from build123d import *

# Parameters (mm, degrees)
ESQUISSE4_W             = 100
ESQUISSE4_H             = 100
ESQUISSE4_W_2           = 90
ESQUISSE4_H_2           = 90
BOSS_EXTRU_1_DEPTH      = 100
ESQUISSE5_W             = 100
ESQUISSE5_H             = 100
BOSS_EXTRU_2_DEPTH      = 10
ESQUISSE6_W             = 95
ESQUISSE6_H             = 94.999780415
ENL_V_MAT_EXTRU_1_DEPTH = 95
ESQUISSE7_W             = 95
ESQUISSE7_H             = 95
ENL_V_MAT_EXTRU_2_DEPTH = 1
ESQUISSE8_W             = 95
ESQUISSE8_H             = 95
BOSS_EXTRU_3_DEPTH      = 1
ENL_V_MAT_EXTRU_4_DEPTH = 55.5
ENL_V_MAT_EXTRU_5_DEPTH = 21.5


with BuildPart() as part:
    # Esquisse4 → Boss.-Extru.1 (new body)
    with BuildSketch(Plane.XY):
        with Locations((1.564199822, -3.801871506)):
            Rectangle(ESQUISSE4_W, ESQUISSE4_H)
        with Locations((1.564199822, -3.801871506)):
            Rectangle(ESQUISSE4_W_2, ESQUISSE4_H_2, mode=Mode.SUBTRACT)
    extrude(amount=BOSS_EXTRU_1_DEPTH)

    # Esquisse5 → Boss.-Extru.2 (add)
    with BuildSketch(Plane.XY.offset(100)):
        with Locations((1.564199822, -3.801871506)):
            Rectangle(ESQUISSE5_W, ESQUISSE5_H)
    extrude(amount=-BOSS_EXTRU_2_DEPTH)

    # Esquisse6 → Enlèv. mat.-Extru.1 (cut)
    with BuildSketch(Plane(origin=(0, 0, 0), x_dir=(-1, 0, 0), z_dir=(0, 0, -1))):
        with Locations((0.935800178, -1.301761713)):
            Rectangle(ESQUISSE6_W, ESQUISSE6_H)
    extrude(amount=-ENL_V_MAT_EXTRU_1_DEPTH, mode=Mode.SUBTRACT)

    # Esquisse7 → Enlèv. mat.-Extru.2 (cut)
    with BuildSketch(Plane(origin=(0, -48.801651921, 0), x_dir=(1, 0, 0), z_dir=(0, 1, 0))):
        with Locations((-0.935800178, -47.5)):
            Rectangle(ESQUISSE7_W, ESQUISSE7_H)
    extrude(amount=-ENL_V_MAT_EXTRU_2_DEPTH, mode=Mode.SUBTRACT)

    # Esquisse8 → Boss.-Extru.3 (add)
    with BuildSketch(Plane(origin=(0, -49.801651921, 0), x_dir=(1, 0, 0), z_dir=(0, 1, 0))):
        with Locations((-0.935800178, -47.5)):
            Rectangle(ESQUISSE8_W, ESQUISSE8_H)
    extrude(amount=BOSS_EXTRU_3_DEPTH)

    # Esquisse9 → Enlèv. mat.-Extru.4 (cut)
    with BuildSketch(Plane(origin=(0, 0, 95), x_dir=(-1, 0, 0), z_dir=(0, 0, -1))):
        with BuildLine():
            ThreePointArc((23.184567711, 20.946945437), (-26.312906972, 20.94700582), (-26.312967355, -28.550468863))
            Line((-26.312967355, -28.550468863), (23.184567711, 20.946945437))
        make_face()
        with BuildLine():
            Line((23.184567711, 20.946945437), (-26.312967355, -28.550468863))
            ThreePointArc((-26.312967355, -28.550468863), (11.829700587, -36.137553521), (33.435800178, -3.801761713))
            ThreePointArc((33.435800178, -3.801761713), (30.771591985, 9.592138696), (23.184567711, 20.946945437))
        make_face()
    extrude(amount=-ENL_V_MAT_EXTRU_4_DEPTH, mode=Mode.SUBTRACT)

    # Esquisse11 → Enlèv. mat.-Extru.5 (cut)
    with BuildSketch(Plane.ZY.offset(-46.564199822)):
        with BuildLine():
            ThreePointArc((25.251232467, 20.946945437), (25.25129285, -28.550529246), (74.748767533, -28.550468863))
            Line((74.748767533, -28.550468863), (25.251232467, 20.946945437))
        make_face()
        with BuildLine():
            Line((25.251232467, 20.946945437), (74.748767533, -28.550468863))
            ThreePointArc((74.748767533, -28.550468863), (82.335791808, -17.195662123), (85, -3.801761713))
            ThreePointArc((85, -3.801761713), (63.393900409, 28.534030094), (25.251232467, 20.946945437))
        make_face()
    extrude(amount=-ENL_V_MAT_EXTRU_5_DEPTH, mode=Mode.SUBTRACT)


solid = part.part
Design review of the part built by this model. Coordinates are the model's own, in mm. A direction names the side the tool comes from. Round coordinates to 2 decimals unless told otherwise and drop trailing zeros. Write each loop counter-clockwise with the first axis right and the second up, starting at its lowest first coordinate (ties: lowest second). Pieces come first, ordered by that corner, then holes.
Item 1: Consider section D-D on x = -35. Give the boundary of the cut face in (y, z), and give its area (3 significant figures).
Item 2: For faces 1 (the flat face through (-2, -48.802, 47)), 2 (the flat face through (-48.436, -26, 98)), list the 3-axis set-ups (+Z, -Z, +X, -X, +Y, -Y) from which the entire face can be reached by the end or side of a thin tool; tool diameter is ignored.
Item 3: Wall thickness on L1, parallel to Z at x = 1.5, y = 31.5; L2, parallel to Y at x = -32.5, z = 37; L3, parallel to X at y = 37, z = 64: over which ranges is each line inside the solid? List them lowest first.
Item 4: Consider section C-C on x = 8. Give the boundary of the cut face in (y, z), and give its area (3 significant figures).
Item 5: Consider section B-B on y = 15. Give the boundary of the cut face in (x, z), and give its area (3 significant figures).
Item 6: For pin 1 Ø3 at (y, z) = (-17, 20.5) entering from -X; pin 2 Ø8 at (x, z) = (-10, 89) entering from +Y; pin 3 Ø12 at (y, z) = (13, 74) entering from -X, all flat-tipped, find the tip position at first contact; note any pin that passes through.
Item 7: Consider section A-A on z = 50. Give the boundary of the cut face in (x, y), and give its area (3 significant figures).
Check values:
1. outline: (-53.8, 0) - (-48.8, 0) - (-48.8, 95) - (46.2, 95) - (46.2, 100) - (-53.8, 100) - close
1. area: 975 mm2
2. face 1: -Z, -X, +Y
2. face 2: +Z, -Z, -X, +Y, -Y
3. L1: z = 95 to 100
3. L2: y = -53.8 to -48.8
3. L3: x = 46.56 to 51.56
4. outline: (-53.8, 0) - (-48.8, 0) - (-48.8, 95) - (-38.2, 95) - (-38.2, 100) - (-53.8, 100) - close; (30.6, 95) - (46.2, 95) - (46.2, 100) - (30.6, 100) - close
4. area: 631 mm2
5. outline: (-48.44, 95) - (-27.96, 95) - (-27.96, 100) - (-48.44, 100) - close; (31.09, 95) - (46.56, 95) - (46.56, 79.52) - (51.56, 79.52) - (51.56, 100) - (31.09, 100) - close; (46.56, 0) - (51.56, 0) - (51.56, 20.48) - (46.56, 20.48) - close
5. area: 385 mm2
6. pin 1: passes through
6. pin 2: stops at y = -48.8
6. pin 3: stops at x = 46.56
7. outline: (-48.44, -53.8) - (51.56, -53.8) - (51.56, -38.8) - (46.56, -38.8) - (46.56, -48.8) - (-48.44, -48.8) - close; (46.56, 31.2) - (51.56, 31.2) - (51.56, 46.2) - (46.56, 46.2) - close
7. area: 625 mm2
